Read the model definition and answer for the solid it produces. Units are mm, in the model's axes. Face numbers are marked on the shaded views. Coordinates: 2 decimals unless noted, no trailing zeros. Order: outer loops, then holes, each group sorted by start corner. A loop starts at its lowest first (then second) coordinate and runs counter-clockwise, first axis right, second up. Notation, with made-up numbers: (29.5, 31.5) -> (76.5, 31.5) arc R6 cw to (76.5, 38.5) -> close; hole circle Ø8 at (11.25, 87.5). An arc over 180 degrees is marked (long way). Answer in a Markdown table with one row per item.
from build123d import *

# Parameters (mm, degrees)
SKETCH1_W           = 53
SKETCH1_H           = 31.5
BOSS_EXTRUDE1_DEPTH = 1.5
SKETCH2_W           = 1.5
SKETCH2_H           = 10
SKETCH2_W_2         = 15
SKETCH2_H_2         = 1.5
BOSS_EXTRUDE2_DEPTH = 4


with BuildPart() as part:
    # Sketch1 → Boss-Extrude1 (new body)
    with BuildSketch(Plane.XY):
        with Locations((26.5, 15.75)):
            Rectangle(SKETCH1_W, SKETCH1_H)
    extrude(amount=BOSS_EXTRUDE1_DEPTH)

    # Sketch2 → Boss-Extrude2 (add)
    with BuildSketch(Plane.XY.offset(1.5)):
        with Locations((0.75, 15.75)):
            Rectangle(SKETCH2_W, SKETCH2_H)
        with Locations((26.5, 30.75)):
            Rectangle(SKETCH2_W_2, SKETCH2_H_2)
        with Locations((52.25, 15.75)):
            Rectangle(SKETCH2_W, SKETCH2_H)
        with Locations((26.5, 0.75)):
            Rectangle(SKETCH2_W_2, SKETCH2_H_2)
    extrude(amount=BOSS_EXTRUDE2_DEPTH)


solid = part.part
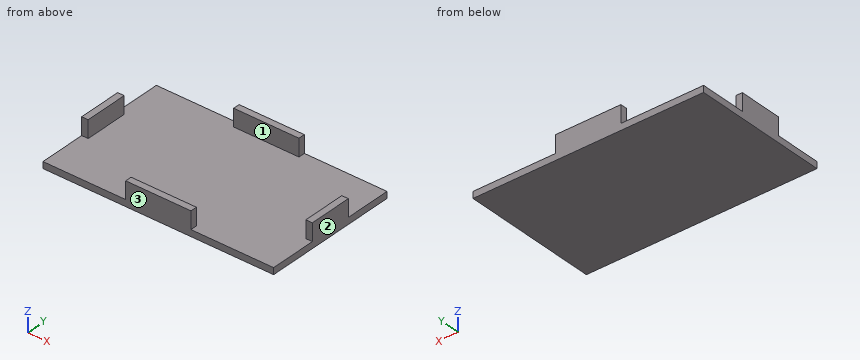
Q1. The part is cut by section A-A (z = 4.4). Write down the section's boundary in (x, y).
Outcome:
| item | result |
|---|---|
| outline | (0, 10.75) -> (1.5, 10.75) -> (1.5, 20.75) -> (0, 20.75) -> close; (19, 0) -> (34, 0) -> (34, 1.5) -> (19, 1.5) -> close; (19, 30) -> (34, 30) -> (34, 31.5) -> (19, 31.5) -> close; (51.5, 10.75) -> (53, 10.75) -> (53, 20.75) -> (51.5, 20.75) -> close |
Q2. The part is cut by section C-C (x = 22). Write down the section's boundary in (y, z), then the cut area to 4 significant figures.
Outcome:
| item | result |
|---|---|
| outline | (0, 0) -> (31.5, 0) -> (31.5, 5.5) -> (30, 5.5) -> (30, 1.5) -> (1.5, 1.5) -> (1.5, 5.5) -> (0, 5.5) -> close |
| area | 59.25 mm² |
Q3. Given pin 1 (1 mm diameter, centred on y = 12.5, z = 0.5, fed in from -X); pin 2 (0.8 mm diameter, centred on x = 52, z = 3.5, fed in from -Y); pin 3 (5 mm diameter, centred on x = 11.5, y = 17, fed in from +Z); pin 4 (0.8 mm diameter, centred on x = 52.5, z = 4, fed in from +Y), each flat-ended and moving along its own axis, determine where each tip first touches the part or whether it passes through.
Outcome:
| item | result |
|---|---|
| pin 1 | x = 0 |
| pin 2 | y = 10.75 |
| pin 3 | z = 1.5 |
| pin 4 | y = 20.75 |
Q4. The part is cut by section D-D (y = 5.5). Write down the section's boundary in (x, z), then the cut area to 3 significant figures.
Outcome:
| item | result |
|---|---|
| outline | (0, 0) -> (53, 0) -> (53, 1.5) -> (0, 1.5) -> close |
| area | 79.5 mm² |
Q5. The part is cut by section B-B (y = 17). Write down the section's boundary in (x, z).
Outcome:
| item | result |
|---|---|
| outline | (0, 0) -> (53, 0) -> (53, 5.5) -> (51.5, 5.5) -> (51.5, 1.5) -> (1.5, 1.5) -> (1.5, 5.5) -> (0, 5.5) -> close |
Q6. Consider line 1 (X direction, y = 20, z = 2.2); line 2 (Y direction, x = 28.5, z = 4.7); line 3 (Z direction, x = 29.5, y = 23). Determine where each line is inside the solid, lowest interval first.
Outcome:
| item | result |
|---|---|
| line 1 | 0 to 1.5, 51.5 to 53 |
| line 2 | 0 to 1.5, 30 to 31.5 |
| line 3 | 0 to 1.5 |
Q7. For a pull along Y with two mould halves and no side action, classify the marked faces 1, 2 and 3 as pulls with the +Y half, pulls with the -Y half, needs draft (parallel to the pull), parting line crosses it, or undercut.
Outcome:
| item | result |
|---|---|
| face 1 | undercut |
| face 2 | needs draft |
| face 3 | pulls with the -Y half |
